Model file for the job. Use its own axes, mm. Face numbers are marked on the shaded views. A direction names the side the tool comes from. Give positions to 0.01 mm unless a question says otherwise; leave off trailing zeros. Loops run counter-clockwise (first coordinate to the right, second up) from the corner with the lowest first, then second, coordinate; pieces in that order, holes last. Notation, with made-up numbers: M 20.25,51 L 50.25,51 A31 cw 50.25,89 Z; hole C -28.5,31.25 d5. An arc over 180 degrees is marked long. Use CSV: the item, a comma, the result in double quotes. Start each with the question number.
(1) Slice it at D-D on y = 90. List the corners of the cut face in (x, z).
(2) Wall check: line 1 along Z through (x, y) = (141.5, 94.5); line 2 along Z through (x, y) = (58, 7); line 3 along Y through (x, z) = (44.5, 117). Give the ranges that are in metal, low to high. Write a range as from..to.
(3) Slice it at B-B on x = 112. List the corners of the cut face in (y, z), and give its area (3 significant figures).
(4) Slice it at A-A on y = 60. List the corners of the cut face in (x, z), and give its area (3 significant figures).
(5) Flat gauge pins, fed straight in: P1, Ø12, axis at y = 67, z = 112, coming from the -X side; P2, Ø2, axis at x = 41, z = 119, coming from the +Y side; P3, Ø3, axis at y = 85, z = 120, coming from the +X side; P4, Ø8, axis at x = 62, y = 19.5, coming from the +Z side. Where does each tip first touch, or does it go through?
(6) Tool access for the marked faces 1 and 2: list every direction of +Z, -Z, +X, -X, +Y, -Y with a clear straight run to the whole face (end or side of a thin tool).
(7) Slice it at C-C on z = 131. List the corners of the cut face in (x, y), and give its area (3 significant figures).
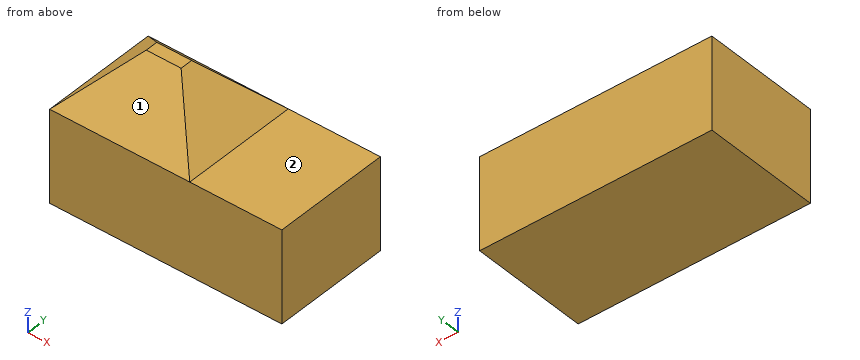
```python
from build123d import *

# Parameters (mm, degrees)
F0_W     = 135.237008
F0_H     = 113.707788
F1_DEPTH = 139.7
F2_SIZE  = 50.8
F3_W     = 113.707788
F3_H     = 88.9
F4_DEPTH = 88.9


with BuildPart() as f1:
    # F0 (on Top) → F1 (new body)
    with BuildSketch(Plane.XY):
        with Locations((67.618504, 56.853894)):
            Rectangle(F0_W, F0_H)
    extrude(amount=F1_DEPTH)

    # F2
    f2_edges = [f1.edges().sort_by_distance(p)[0] for p in [
        (0, 56.853894, 139.7),
        (67.618504, 0, 139.7),
        (135.237008, 56.853894, 139.7),
        (67.618504, 113.707788, 139.7),
    ]]
    chamfer(f2_edges, length=F2_SIZE)

    # F3 (on face) → F4 (join)
    with BuildSketch(Plane.YZ.offset(135.237008)):
        with Locations((56.853894, 44.45)):
            Rectangle(F3_W, F3_H)
    extrude(amount=F4_DEPTH)


solid = f1.part
```
Reply:
1,outline,"M 0,0 L 224.14,0 L 224.14,88.9 L 135.24,88.9 L 111.53,112.61 L 23.71,112.61 L 0,88.9 Z"
2,line 1,"z = 0..88.9"
2,line 2,"z = 0..95.9"
2,line 3,"y = 28.1..85.61"
3,outline,"M 0,0 L 113.71,0 L 113.71,88.9 L 90.47,112.14 L 23.24,112.14 L 0,88.9 Z"
3,area,"12,200 mm^2"
4,outline,"M 0,0 L 224.14,0 L 224.14,88.9 L 135.24,88.9 L 84.44,139.7 L 50.8,139.7 L 0,88.9 Z"
4,area,"24,200 mm^2"
5,P1,"stops at x = 17.1"
5,P2,"stops at y = 84.61"
5,P3,"passes through"
5,P4,"stops at z = 112.4"
6,face 1,"+Z, +X, -X, -Y"
6,face 2,"+Z, +X, +Y, -Y"
7,outline,"M 42.1,42.1 L 93.14,42.1 L 93.14,71.61 L 42.1,71.61 Z"
7,area,"1,510 mm^2"
